Geometry: final body of the model. Coordinates: model frame, mm. A direction names the side the tool comes from. Give positions to 0.01 mm unless a question says otherwise; leave off trailing zeros. Order: outer loops, then holes, each group sorted by start corner. A loop starts at its lowest first (then second) coordinate and runs counter-clockwise, first axis right, second up. Notation, with made-up numbers: (-9, 49.5) - (19, 49.5) arc R26 cw to (19, 70.5) - close; hole circle Ø7 at (-38.5, 13.25). An arc over 180 degrees is marked (long way). Use one line per item in the form item = value.
from build123d import *

# Parameters (mm, degrees)
F1_DEPTH  = 38.1
F2_R      = 9.0076691871
F3_DEPTH  = 18.4852466609
F4_R      = 11.43
F4_R_2    = 9.0076691871
F6_DEPTH  = 9.398
F7_DEPTH  = 25.4
F10_DEPTH = 5.715
F12_R     = 25.4
F13_R     = 12.7
F14_R     = 1.27


# Not quite as in the source:
# - a pattern or mirror of a feature is missing from the dataset's text; its kind, count and spacing are read off the source's solid


with BuildPart() as f1:
    # F0 (on Front) → F1 (new body, symmetric)
    with BuildSketch(Plane.XZ):
        Polygon((0, 0), (0, 74.0791857243), (-18.4852466609, 74.0791857243), (-18.4852466609, 14.5855043083), (-59.9480941892, 14.5855043083), (-59.9480941892, 0), align=None)
    extrude(amount=F1_DEPTH, both=True)

    # F2 (on face) → F3 (cut, through all)
    with BuildSketch(Plane(origin=(-18.4852466609, 0, 0), x_dir=(0, -1, 0), z_dir=(-1, 0, 0))):
        with Locations((0, 61.3791857243)):
            Circle(F2_R)
    extrude(amount=-F3_DEPTH, mode=Mode.SUBTRACT)

    # F4 (on face) → F6 (cut)
    with BuildSketch(Plane(origin=(-18.4852466609, 0, 0), x_dir=(0, -1, 0), z_dir=(-1, 0, 0))):
        with Locations((0, 61.3791857243)):
            Circle(F4_R)
        with Locations((0, 61.3791857243)):
            Circle(F4_R_2, mode=Mode.SUBTRACT)
    extrude(amount=-F6_DEPTH, mode=Mode.SUBTRACT)

    # F5 (on face) → F7 (cut)
    with BuildSketch(Plane.XY.offset(14.5855043083)):
        with BuildLine():
            ThreePointArc((-47.9387399794, -8.003022201), (-55.2808618291, 0), (-47.9387399794, 8.003022201))
            Line((-47.9387399794, 8.003022201), (-59.9480941892, 8.003022201))
            Line((-59.9480941892, 8.003022201), (-59.9480941892, -8.003022201))
            Line((-59.9480941892, -8.003022201), (-47.9387399794, -8.003022201))
        make_face()
        with BuildLine():
            ThreePointArc((-47.9387399794, -8.003022201), (-41.8177369816, -5.9191702591), (-39.2153265492, 0))
            ThreePointArc((-39.2153265492, 0), (-41.8177369816, 5.9191702591), (-47.9387399794, 8.003022201))
            ThreePointArc((-47.9387399794, 8.003022201), (-55.2808618291, 0), (-47.9387399794, -8.003022201))
        make_face()
    extrude(amount=-F7_DEPTH, mode=Mode.SUBTRACT)

    # F9 (on offset) → F10 (join, symmetric)
    with BuildSketch(Plane.XZ.offset(25.4)):
        Polygon((-41.8496876955, 14.5855043083), (-18.4852466609, 14.5855043083), (-18.4852466609, 44.3323450163), align=None)
    f10 = extrude(amount=F10_DEPTH, both=True)

    # F10_copies: F10 across plane
    add(f10.mirror(Plane.ZX))

    # F12
    f12_edges = [f1.edges().sort_by_distance(p)[0] for p in [
        (-9.242623, 38.1, 74.079186),
        (-9.242623, -38.1, 74.079186),
    ]]
    fillet(f12_edges, radius=F12_R)

    # F13
    f13_edges = [f1.edges().sort_by_distance(p)[0] for p in [
        (0, 0, 0),
    ]]
    fillet(f13_edges, radius=F13_R)

    # F14
    f14_edges = [f1.edges().sort_by_distance(p)[0] for p in [
        (0, 38.1, 30.689593),
        (0, 0, 12.7),
        (0, 30.660512, 66.639698),
        (0, -38.1, 30.689593),
        (0, 0, 74.079186),
        (0, -30.660512, 66.639698),
        (0, 9.007669, 61.379186),
        (-59.948094, 23.051511, 0),
        (-3.719744, 38.1, 3.719744),
        (-36.324047, 38.1, 0),
        (-3.719744, -38.1, 3.719744),
        (-36.324047, -38.1, 0),
        (-59.948094, -38.1, 7.292752),
        (-59.948094, -23.051511, 0),
        (-59.948094, 8.003022, 7.292752),
        (-59.948094, -23.051511, 14.585504),
        (-59.948094, -8.003022, 7.292752),
    ]]
    fillet(f14_edges, radius=F14_R)


solid = f1.part
(1) Ray query, line 1 along Z through (x, y) = (-15, 0); line 2 along X through (y, z) = (-8, 48); line 3 along Y through (x, z) = (-25, 33.5) (3 decimals). Return the intervals inside material, ascending.
Computed values:
line_1 = 0 to 49.95, 72.81 to 74.08
line_2 = -18.49 to 0
line_3 = -31.115 to -19.685, 19.685 to 31.115
(2) Cut plane A-A on z = 20. Output: boundary loops of the cut face in (x, y) (3 decimals), plus the area to 3 significant figures.
Computed values:
outline = (-37.597, -31.115) - (-18.485, -31.115) - (-18.485, -38.1) - (-1.27, -38.1) arc R1.27 ccw to (0, -36.83) - (0, 36.83) arc R1.27 ccw to (-1.27, 38.1) - (-18.485, 38.1) - (-18.485, 31.115) - (-37.597, 31.115) - (-37.597, 19.685) - (-18.485, 19.685) - (-18.485, -19.685) - (-37.597, -19.685) - close
area = 1,840 mm²
(3) Pull-direction query (Y, two-part tool) for faces 4 (the face through (-18, 38.1, 20)), 5 (the face through (-30, -25.48, 29.67)), 6 (the face through (-25, 19.685, 23)); classes: released by +Y, released by -Y, zero draft, split by the parting line, or undercut.
Computed values:
face_4 = released by +Y
face_5 = zero draft
face_6 = undercut
(4) Cut plane C-C on x = -35. Output: boundary loops of the cut face in (y, z) (1 decimal).
Computed values:
outline = (-38.1, 1.3) arc R1.3 ccw to (-36.8, 0) - (36.8, 0) arc R1.3 ccw to (38.1, 1.3) - (38.1, 14.6) - (31.1, 14.6) - (31.1, 23.3) - (19.7, 23.3) - (19.7, 14.6) - (-19.7, 14.6) - (-19.7, 23.3) - (-31.1, 23.3) - (-31.1, 14.6) - (-38.1, 14.6) - close
(5) Reachability of faces 1 (the face through (-9.087, 9, 58)), 2 (the face through (-53, -8.003, 7)), 3 (the face through (-25, -31.115, 23)) from +Z, -Z, +X, -X, +Y, -Y: full face, straight path, thin tool, end or side. Return the list, or none.
Computed values:
face_1 = -X
face_2 = +Z, -Z, -X
face_3 = +Z, -X, -Y
(6) Cut plane B-B on x = -45.5. Output: boundary loops of the cut face in (y, z), plus the area to 3 significant figures.
Computed values:
outline = (-38.1, 1.27) arc R1.27 ccw to (-36.83, 0) - (-7.84, 0) - (-7.84, 14.59) - (-38.1, 14.59) - close; (7.84, 0) - (36.83, 0) arc R1.27 ccw to (38.1, 1.27) - (38.1, 14.59) - (7.84, 14.59) - close
area = 882 mm²
(7) Contact query for flat-ended pins moving along their axis: pin 1 Ø25 at (y, z) = (4.5, 60) entering from -X; pin 2 Ø1.5 at (x, z) = (-28, 23.5) entering from -Y (3 decimals); pin 3 Ø10 at (y, z) = (30, 55) entering from +X; pin 4 Ø11.5 at (x, z) = (-27, 27) entering from +Y (3 decimals). Output: stop coordinate, or through.
Computed values:
pin_1 = -18.49
pin_2 = -31.115
pin_3 = 0
pin_4 = 31.115
